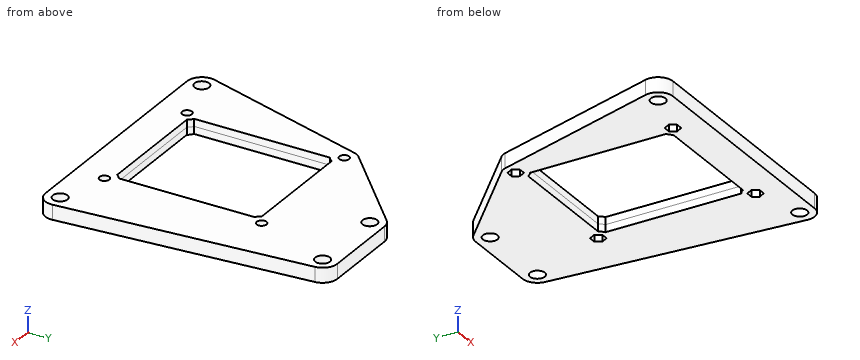
```python
from build123d import *

# Parameters (mm, degrees)
SKETCH001_R    = 1.5
SKETCH001_R_2  = 1
PAD_DEPTH      = 1.5
PAD_DEPTH_BACK = 1.5
SKETCH002_R    = 1
POCKET_DEPTH   = 2


with BuildPart() as part:
    # Sketch001 → Pad (new body, two sides)
    with BuildSketch(Plane.XY) as pad_sk:
        with BuildLine():
            Line((26.990815, -15.765426), (22.990815, 35.234574))
            ThreePointArc((22.990815, 35.234574), (22.036698, 37.202694), (20, 38))
            Line((20, 38), (4, 38))
            ThreePointArc((4, 38), (2.904805, 37.792946), (1.960786, 37.200365))
            Line((1.960786, 37.200365), (-15.699328, 20.833653))
            ThreePointArc((-15.699328, 20.833653), (-16.121162, 20.323129), (-16.394149, 19.719757))
            Line((-26.872979, -15.136292), (-16.394149, 19.719757))
            ThreePointArc((-26.872979, -15.136292), (-26.407397, -17.790094), (-24, -19))
            Line((-24, -19), (24, -19))
            ThreePointArc((24, -19), (26.202694, -18.036698), (26.990815, -15.765426))
        make_face()
        with Locations((20, 35)):
            Circle(SKETCH001_R, mode=Mode.SUBTRACT)
        with Locations((4, 35)):
            Circle(SKETCH001_R, mode=Mode.SUBTRACT)
        with Locations((-24, -16)):
            Circle(SKETCH001_R, mode=Mode.SUBTRACT)
        with Locations((24, -16)):
            Circle(SKETCH001_R, mode=Mode.SUBTRACT)
        with Locations((-14, 19)):
            Circle(SKETCH001_R_2, mode=Mode.SUBTRACT)
        with Locations((14, 19)):
            Circle(SKETCH001_R_2, mode=Mode.SUBTRACT)
        with Locations((-14, -13)):
            Circle(SKETCH001_R_2, mode=Mode.SUBTRACT)
        with Locations((14, -13)):
            Circle(SKETCH001_R_2, mode=Mode.SUBTRACT)
        with BuildLine():
            ThreePointArc((-12.75, 16.834936), (-12.232233, 17.232233), (-11.834936, 17.75))
            Line((-11.834936, 17.75), (11.834936, 17.75))
            ThreePointArc((11.834936, 17.75), (12.232233, 17.232233), (12.75, 16.834936))
            Line((12.75, 16.834936), (12.75, -10.834936))
            ThreePointArc((12.75, -10.834936), (12.232233, -11.232233), (11.834936, -11.75))
            Line((-11.834936, -11.75), (11.834936, -11.75))
            ThreePointArc((-11.834936, -11.75), (-12.232233, -11.232233), (-12.75, -10.834936))
            Line((-12.75, -10.834936), (-12.75, 16.834936))
        make_face(mode=Mode.SUBTRACT)
    extrude(amount=PAD_DEPTH)
    extrude(pad_sk.sketch, amount=-PAD_DEPTH_BACK)

    # Sketch002 → Pocket (cut)
    with BuildSketch(Plane.XY):
        Polygon((-13.278312, -14.25), (-12.556624, -13), (-13.278312, -11.75), (-14.721688, -11.75), (-15.443376, -13), (-14.721688, -14.25), align=None)
        with Locations((-14, -13)):
            Circle(SKETCH002_R, mode=Mode.SUBTRACT)
        Polygon((14.721688, -14.25), (15.443376, -13), (14.721688, -11.75), (13.278312, -11.75), (12.556624, -13), (13.278312, -14.25), align=None)
        with Locations((14, -13)):
            Circle(SKETCH002_R, mode=Mode.SUBTRACT)
        Polygon((14.721688, 17.75), (15.443376, 19), (14.721688, 20.25), (13.278312, 20.25), (12.556624, 19), (13.278312, 17.75), align=None)
        with Locations((14, 19)):
            Circle(SKETCH002_R, mode=Mode.SUBTRACT)
        Polygon((-13.278312, 17.75), (-12.556624, 19), (-13.278312, 20.25), (-14.721688, 20.25), (-15.443376, 19), (-14.721688, 17.75), align=None)
        with Locations((-14, 19)):
            Circle(SKETCH002_R, mode=Mode.SUBTRACT)
    extrude(amount=-POCKET_DEPTH, mode=Mode.SUBTRACT)


solid = part.part
```
Geometry: final body of the model. Coordinates: model frame, mm. Round coordinates to 2 decimals unless told otherwise and drop trailing zeros. Loops run counter-clockwise (first coordinate to the right, second up) from the corner with the lowest first, then second, coordinate; pieces in that order, holes last.
Item 1: Section B-B, the plane y = 3.5. Output: boundary loops of the cut face in (x, z), plus the area to 3 significant figures.
Checked values:
outline: (-21.27, -1.5) - (-12.75, -1.5) - (-12.75, 1.5) - (-21.27, 1.5) - close; (12.75, -1.5) - (25.48, -1.5) - (25.48, 1.5) - (12.75, 1.5) - close
area: 63.8 mm2
Item 2: Line query: L1, parallel to Y at x = 4, z = -0.35; L2, parallel to Y at x = 9, z = 1.3; L3, parallel to Y at x = -13, z = -1.05. Output: solid intervals per line, ascending.
Checked values:
L1: y = -19 to -11.75, 17.75 to 33.5, 36.5 to 38
L2: y = -19 to -11.75, 17.75 to 38
L3: y = -19 to -13.77, -12.23 to 18.23, 19.77 to 23.34
Item 3: Contact query for flat-ended pins moving along their axis: P1, Ø1, axis at y = 3, z = 0.5, coming from the +X side; P2, Ø1, axis at y = 6.5, z = 1, coming from the +X side; P3, Ø0.8, axis at y = -2.5, z = -1, coming from the +X side. Output: stop coordinate, or through.
Checked values:
P1: stops at x = 25.56
P2: stops at x = 25.28
P3: stops at x = 25.98
Item 4: Section C-C, the plane z = 1.05. State how many separate pieces and enclosed holes the cut face has, plus the area to 3 significant figures.
Checked values:
separate pieces: 1
enclosed holes: 9
area: 1,620 mm2
Item 5: Section D-D, the plane y = -2.5. Output: boundary loops of the cut face in (x, z), plus the area to 3 significant figures.
Checked values:
outline: (-23.07, -1.5) - (-12.75, -1.5) - (-12.75, 1.5) - (-23.07, 1.5) - close; (12.75, -1.5) - (25.95, -1.5) - (25.95, 1.5) - (12.75, 1.5) - close
area: 70.6 mm2
Item 6: Section A-A, the plane x = 14. Output: boundary loops of the cut face in (y, z).
Checked values:
outline: (-19, -1.5) - (-14.25, -1.5) - (-14.25, 0) - (-14, 0) - (-14, 1.5) - (-19, 1.5) - close; (-12, 0) - (-11.75, 0) - (-11.75, -1.5) - (17.75, -1.5) - (17.75, 0) - (18, 0) - (18, 1.5) - (-12, 1.5) - close; (20, 0) - (20.25, 0) - (20.25, -1.5) - (38, -1.5) - (38, 1.5) - (20, 1.5) - close
